Source: CAD feature listing. Evaluate the final solid. Frame: model axes, mm. Face numbers are marked on the shaded views. A direction names the side the tool comes from. Give positions to 0.01 mm unless a question says otherwise; leave off trailing zeros. Order: outer loops, then holes, each group sorted by start corner. A loop starts at its lowest first (then second) coordinate and runs counter-clockwise, first axis right, second up. Notation, with made-up numbers: M 72,37 L 101,37 A27 cw 101,56 Z; hole C -22.75,43 d10. An arc over 180 degrees is marked long. Answer in a Markdown table with one row per item. Add a question column.
(1) Set-up query: the marked faces 4, 5 and 6. Return all of +Z, -Z, +X, -X, +Y, -Y with unobstructed straight access to the full face (end or side cutting, diameter ignored); none if empty.
(2) Section query C-C, the plane x = -6.5. Return loops of the section in (y, z).
(3) Section query B-B, the plane z = 4.45. Return loops of the section in (x, y), plus the area to 3 significant figures.
(4) Pin query (flat end, axial travel): P1, Ø2, axis at y = -11.5, z = 4, coming from the -X side; P2, Ø1.5, axis at y = -9, z = 1.5, coming from the +X side; P3, Ø4, axis at x = -3, y = 3.5, coming from the -Z side; P4, Ø10, axis at x = -10.5, y = -6.5, coming from the -Z side. Return the tip coordinate at first contact, or that it passes through.
(5) Section query D-D, the plane x = 5.5. Return loops of the section in (y, z), plus the area to 3 significant figures.
(6) Mould query, pull axis Y, two halves, no side actions, for the marked faces 1, 2 and 3. Classes: pulls with the +Y half, pulls with the -Y half, needs draft (parallel to the pull), parting line crosses it, or undercut.
(7) Material intervals for line 1 along X through (y, z) = (-12, 4.7); line 2 along X through (y, z) = (-0.25, 1.6); line 3 along Y through (x, z) = (-6.5, 1.65), sorted ascending.
(8) Section query A-A, the plane y = -10. Return loops of the section in (x, z).
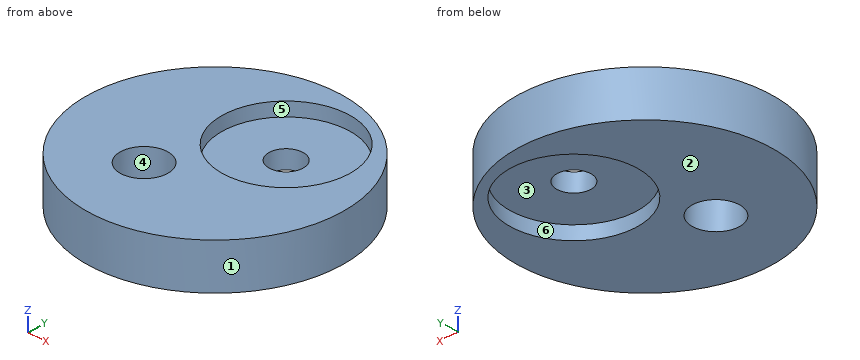
from build123d import *

# Parameters (mm, degrees)
ESQUISSE1_R             = 14
ESQUISSE1_R_2           = 1.874597255
ESQUISSE1_R_3           = 2.6
BOSS_EXTRU_1_DEPTH      = 5
ESQUISSE2_R             = 7
ENL_V_MAT_EXTRU_1_DEPTH = 1.5
ESQUISSE3_R             = 7
ENL_V_MAT_EXTRU_2_DEPTH = 1.5


with BuildPart() as part:
    # Esquisse1 → Boss.-Extru.1 (new body)
    with BuildSketch(Plane.XY):
        with Locations((-3.25, -5)):
            Circle(ESQUISSE1_R)
        Circle(ESQUISSE1_R_2, mode=Mode.SUBTRACT)
        with Locations((-6.5, -10)):
            Circle(ESQUISSE1_R_3, mode=Mode.SUBTRACT)
    extrude(amount=BOSS_EXTRU_1_DEPTH)

    # Esquisse2 → Enlèv. mat.-Extru.1 (cut)
    with BuildSketch(Plane.XY.offset(5)):
        Circle(ESQUISSE2_R)
    extrude(amount=-ENL_V_MAT_EXTRU_1_DEPTH, mode=Mode.SUBTRACT)

    # Esquisse3 → Enlèv. mat.-Extru.2 (cut)
    with BuildSketch(Plane(origin=(0, 0, 0), x_dir=(-1, 0, 0), z_dir=(0, 0, -1))):
        Circle(ESQUISSE3_R)
    extrude(amount=-ENL_V_MAT_EXTRU_2_DEPTH, mode=Mode.SUBTRACT)


solid = part.part
Values follow:
| question | item | result |
|---|---|---|
| 1 | face 4 | +Z, -Z |
| 1 | face 5 | +Z |
| 1 | face 6 | -Z |
| 2 | outline | M -18.62,0 L -12.6,0 L -12.6,5 L -18.62,5 Z; M -7.4,0 L -2.6,0 L -2.6,1.5 L 2.6,1.5 L 2.6,0 L 8.62,0 L 8.62,5 L 2.6,5 L 2.6,3.5 L -2.6,3.5 L -2.6,5 L -7.4,5 Z |
| 3 | outline | C -3.25,-5 d28; hole C -6.5,-10 d5.2; hole C 0,0 d14 |
| 3 | area | 441 mm² |
| 4 | P1 | stops at x = -16.12 |
| 4 | P2 | stops at x = 10.37 |
| 4 | P3 | stops at z = 1.5 |
| 4 | P4 | stops at z = 0 |
| 5 | outline | M -15.93,0 L -4.33,0 L -4.33,1.5 L 4.33,1.5 L 4.33,0 L 5.93,0 L 5.93,5 L 4.33,5 L 4.33,3.5 L -4.33,3.5 L -4.33,5 L -15.93,5 Z |
| 5 | area | 83.3 mm² |
| 6 | face 1 | parting line crosses it |
| 6 | face 2 | needs draft |
| 6 | face 3 | undercut |
| 7 | line 1 | x = -15.37 to -8.16, -4.84 to 8.87 |
| 7 | line 2 | x = -16.42 to -1.86, 1.86 to 9.92 |
| 7 | line 3 | y = -18.62 to -12.6, -7.4 to 8.62 |
| 8 | outline | M -16.33,0 L -9.1,0 L -9.1,5 L -16.33,5 Z; M -3.9,0 L 9.83,0 L 9.83,5 L -3.9,5 Z |
